```python
from build123d import *

# Parameters (mm, degrees)
SKETCH1_W           = 180
SKETCH1_H           = 40
BOSS_EXTRUDE1_DEPTH = 56
SKETCH2_W           = 150
SKETCH2_H           = 10
CUT_EXTRUDE1_DEPTH  = 40
SKETCH3_R           = 25
BOSS_EXTRUDE2_DEPTH = 24.5
BOSS_EXTRUDE3_START = -13.5
SKETCH4_R           = 25
BOSS_EXTRUDE3_DEPTH = 13.5
SKETCH6_R           = 12.5
CUT_EXTRUDE2_DEPTH  = 90
SKETCH10_W          = 11.29862099
SKETCH10_H          = 40
CUT_EXTRUDE4_DEPTH  = 52
SKETCH11_W          = 52
SKETCH11_H          = 40
CUT_EXTRUDE5_DEPTH  = 2
FILLET1_R           = 20


with BuildPart() as part:
    # Sketch1 → Boss-Extrude1 (new body)
    with BuildSketch(Plane.XY):
        with Locations((90, 20)):
            Rectangle(SKETCH1_W, SKETCH1_H)
    extrude(amount=BOSS_EXTRUDE1_DEPTH)

    # Sketch2 → Cut-Extrude1 (cut)
    with BuildSketch(Plane(origin=(0, 0, 0), x_dir=(-1, 0, 0), z_dir=(0, 0, -1))):
        with Locations((-90, 20)):
            Rectangle(SKETCH2_W, SKETCH2_H)
    extrude(amount=-CUT_EXTRUDE1_DEPTH, mode=Mode.SUBTRACT)

    # Sketch3 → Boss-Extrude2 (add)
    with BuildSketch(Plane(origin=(90, 0, 0), x_dir=(0, 0, -1), z_dir=(1, 0, 0))):
        with Locations((-70, 20)):
            Circle(SKETCH3_R)
    boss_extrude2 = extrude(amount=BOSS_EXTRUDE2_DEPTH)

    # Sketch4 → Boss-Extrude3 (add)
    with BuildSketch(Plane(origin=(180, 0, 0), x_dir=(0, 0, -1), z_dir=(1, 0, 0)).offset(BOSS_EXTRUDE3_START)):
        with Locations((-70, 20)):
            Circle(SKETCH4_R)
    boss_extrude3 = extrude(amount=BOSS_EXTRUDE3_DEPTH)

    # Sketch6 → Cut-Extrude2 (cut)
    with BuildSketch(Plane(origin=(180, 0, 0), x_dir=(0, 0, -1), z_dir=(1, 0, 0))):
        with Locations((-70, 20)):
            Circle(SKETCH6_R)
    cut_extrude2 = extrude(amount=-CUT_EXTRUDE2_DEPTH, mode=Mode.SUBTRACT)

    # Mirror1: Boss-Extrude2, Boss-Extrude3, Cut-Extrude2 across plane
    add(boss_extrude2.mirror(Plane(origin=(90, 0, 0), x_dir=(0, 0, 1), z_dir=(1, 0, 0))))
    add(boss_extrude3.mirror(Plane(origin=(90, 0, 0), x_dir=(0, 0, 1), z_dir=(1, 0, 0))))
    add(cut_extrude2.mirror(Plane(origin=(90, 0, 0), x_dir=(0, 0, 1), z_dir=(1, 0, 0))), mode=Mode.SUBTRACT)

    # Sketch10 → Cut-Extrude4 (cut)
    with BuildSketch(Plane(origin=(114.5, 0, 0), x_dir=(0, 0, -1), z_dir=(1, 0, 0))):
        with Locations((-49.350689505, 20)):
            Rectangle(SKETCH10_W, SKETCH10_H)
    cut_extrude4 = extrude(amount=CUT_EXTRUDE4_DEPTH, mode=Mode.SUBTRACT)

    # Mirror3: Cut-Extrude4 across plane
    add(cut_extrude4.mirror(Plane(origin=(90, 0, 0), x_dir=(0, 0, 1), z_dir=(1, 0, 0))), mode=Mode.SUBTRACT)

    # Sketch11 → Cut-Extrude5 (cut)
    with BuildSketch(Plane.XY.offset(56)):
        with Locations((140.5, 20)):
            Rectangle(SKETCH11_W, SKETCH11_H)
    cut_extrude5 = extrude(amount=-CUT_EXTRUDE5_DEPTH, mode=Mode.SUBTRACT)

    # Mirror4: Cut-Extrude5 across plane
    add(cut_extrude5.mirror(Plane(origin=(90, 0, 0), x_dir=(0, 0, 1), z_dir=(1, 0, 0))), mode=Mode.SUBTRACT)

    # Fillet1
    fillet1_edges = [part.edges().sort_by_distance(p)[0] for p in [
        (39.5, 40, 43.70137901),
        (39.5, 0, 43.70137901),
        (140.5, 40, 43.70137901),
        (140.5, 0, 43.70137901),
    ]]
    fillet(fillet1_edges, radius=FILLET1_R - 0.0001)  # a hair under: the kernel refuses the full size


solid = part.part
```
For this review, take the finished solid that the model builds, in its own axes (mm). A direction names the side the tool comes from. Give positions to 0.01 mm unless a question says otherwise; leave off trailing zeros. Write each loop counter-clockwise with the first axis right and the second up, starting at its lowest first coordinate (ties: lowest second). Pieces come first, ordered by that corner, then holes.
Item 1: Insertion check: P1, Ø3, axis at x = 60, y = 19.5, coming from the -Z side; P2, Ø6, axis at x = 30.5, z = 17, coming from the +Y side; P3, Ø1.5, axis at x = 157, z = 46, coming from the +Y side (1 decimal); P4, Ø1, axis at x = 87, z = 78.5, coming from the -Y side. Each pin has a flat end and moves straight along its axis. Give the tip position at first contact, or say it passes through.
Item 2: Wall thickness on probe 1 along X at (y, z) = (19.5, 85); probe 2 along Y at (x, z) = (58.5, 14.5); probe 3 along X at (y, z) = (24, 37.5): over which ranges is each line inside the solid? List them lowest first.
Item 3: Take a section at C-C (z = 85). Give the boundary of the cut face in (x, y).
Item 4: Machinability: for faces 4 (the face through (91, 20, 40)), 5 (the face through (140.864, 33.986, 37.998)), 6 (the face through (39.136, 6.014, 37.998)), which of the approach directions +Z, -Z, +X, -X, +Y, -Y give a long, thin tool a straight path to every point of the face, cutting with its end or side? Answer none if there is none.
Item 5: Take a section at D-D (x = 100.5). Give the boundary of the cut face in (y, z).
Item 6: The part is to be moulded in two halves that separate along X. For faces 1 (the face through (173.16, 20.77, 94.99)), 2 (the face through (0, 20, 47)), 3 (the face through (91, 25, 20)), say which applies: +X half, -X half, draft (parallel to the pull), parting line (faces both ways), or undercut.
Item 7: Take a section at A-A (z = 70). Give the boundary of the cut face in (x, y), and give its area (3 significant figures).
Established:
1. P1: stops at z = 40
1. P2: stops at y = 40
1. P3: passes through
1. P4: stops at y = -3.69
2. probe 1: x = 0 to 13.5, 65.5 to 114.5, 166.5 to 180
2. probe 2: y = 0 to 15, 25 to 40
2. probe 3: x = 0 to 15, 165 to 180
3. outline: (0, 0) - (13.5, 0) - (13.5, 40) - (0, 40) - close; (65.5, 0) - (114.5, 0) - (114.5, 40) - (65.5, 40) - close; (166.5, 0) - (180, 0) - (180, 40) - (166.5, 40) - close
4. face 4: -Z
4. face 5: +Z, +Y
4. face 6: +Z, -Y
5. outline: (0, 0) - (15, 0) - (15, 40) - (25, 40) - (25, 0) - (40, 0) - (40, 55) arc R25 ccw (long way) to (0, 55) - close; hole circle Ø25 at (20, 70)
6. face 1: draft
6. face 2: -X half
6. face 3: undercut
7. outline: (0, -5) - (13.5, -5) - (13.5, 7.5) - (0, 7.5) - close; (0, 32.5) - (13.5, 32.5) - (13.5, 45) - (0, 45) - close; (65.5, -5) - (114.5, -5) - (114.5, 7.5) - (65.5, 7.5) - close; (65.5, 32.5) - (114.5, 32.5) - (114.5, 45) - (65.5, 45) - close; (166.5, -5) - (180, -5) - (180, 7.5) - (166.5, 7.5) - close; (166.5, 32.5) - (180, 32.5) - (180, 45) - (166.5, 45) - close
7. area: 1,900 mm2
